from build123d import *

# Parameters (mm, degrees)
F0_W     = 9.2
F0_H     = 5
F1_DEPTH = 8
F3_R     = 0.75
F6_DEPTH = 30
F7_DEPTH = 4.2
F8_DEPTH = 25


with BuildPart() as f1:
    # F0 (on Front) → F1 (new body, symmetric)
    with BuildSketch(Plane.XZ):
        Polygon((-6, -2.5), (-4.6, -2.5), (-4.6, 2.5), align=None)
        Rectangle(F0_W, F0_H)
        Polygon((4.6, -2.5), (6, -2.5), (4.6, 2.5), align=None)
    extrude(amount=F1_DEPTH, both=True)

    # F3
    f3_edges = [f1.edges().sort_by_distance(p)[0] for p in [
        (-4.6, 0, 2.5),
        (4.6, 0, 2.5),
        (6, 0, -2.5),
        (-6, 0, -2.5),
    ]]
    fillet(f3_edges, radius=F3_R)

    # F5 (on face) → F6 (cut)
    with BuildSketch(Plane.XZ.offset(8)):
        with BuildLine():
            Line((7.368007, 1), (7.368007, 4))
            Line((7.368007, 4), (-7.368007, 4))
            Line((-7.368007, 4), (-7.368007, 1))
            Line((-7.368007, 1), (-5.02, 1))
            Line((-5.02, 1), (-4.753378, 1.952222))
            ThreePointArc((-4.753378, 1.952222), (-4.484384, 2.347565), (-4.031155, 2.5))
            Line((-4.031155, 2.5), (4.031155, 2.5))
            ThreePointArc((4.031155, 2.5), (4.484384, 2.347565), (4.753378, 1.952222))
            Line((4.753378, 1.952222), (5.02, 1))
            Line((5.02, 1), (7.368007, 1))
        make_face()
        with BuildLine():
            Line((-5.02, 1), (5.02, 1))
            Line((5.02, 1), (4.753378, 1.952222))
            ThreePointArc((4.753378, 1.952222), (4.484384, 2.347565), (4.031155, 2.5))
            Line((4.031155, 2.5), (-4.031155, 2.5))
            ThreePointArc((-4.031155, 2.5), (-4.484384, 2.347565), (-4.753378, 1.952222))
            Line((-4.753378, 1.952222), (-5.02, 1))
        make_face()
    extrude(amount=-F6_DEPTH, mode=Mode.SUBTRACT)

    # F4 (on face) → F7 (cut)
    with BuildSketch(Plane.XY.offset(2.5)):
        Polygon((3.95, -2.280534), (3.95, 2.280534), (0, 4.561067), (-3.95, 2.280534), (-3.95, -2.280534), (0, -4.561067), align=None)
    extrude(amount=-F7_DEPTH, mode=Mode.SUBTRACT)

    # F2 (on face) → F8 (cut)
    with BuildSketch(Plane(origin=(0, 0, -2.5), x_dir=(1, 0, 0), z_dir=(0, 0, -1))):
        with BuildLine():
            Line((0, -2), (0, 0))
            Line((0, 0), (0, 2))
            ThreePointArc((0, 2), (-2, 0), (0, -2))
        make_face()
        with BuildLine():
            Line((0, 2), (0, 0))
            Line((0, 0), (0, -2))
            ThreePointArc((0, -2), (1.414214, -1.414214), (2, 0))
            ThreePointArc((2, 0), (1.414214, 1.414214), (0, 2))
        make_face()
    extrude(amount=-F8_DEPTH, mode=Mode.SUBTRACT)


solid = f1.part
Input: part model. Units: mm. Frame: model coordinates. A direction names the side the tool comes from. Round coordinates to 2 decimals unless told otherwise and drop trailing zeros. Order: outer loops, then holes, each group sorted by start corner. A loop starts at its lowest first (then second) coordinate and runs counter-clockwise, first axis right, second up. Notation, with made-up numbers: (78, -29) - (132, -29) arc R20 cw to (132, -9) - close; hole circle Ø7 at (51, 42.5). An arc over 180 degrees is marked (long way). Use a Markdown table: item, result.
1. Mould query, pull axis Y, two halves, no side actions, for faces 1 (the face through (-1.947, 3.437, -0.331)), 2 (the face through (0, 8, -1)), 3 (the face through (-5.372, -0.112, -0.256)). Classes: +Y half, -Y half, draft (parallel to the pull), parting line (faces both ways), or undercut.
Evaluation:
| item | result |
|---|---|
| face 1 | undercut |
| face 2 | +Y half |
| face 3 | draft |
2. Section A-A on x = -1.75. Return the cut outline in (y, z).
Evaluation:
| item | result |
|---|---|
| outline | (-8, -2.5) - (-0.97, -2.5) - (-0.97, -1.7) - (-3.55, -1.7) - (-3.55, 1) - (-8, 1) - close; (0.97, -2.5) - (8, -2.5) - (8, 1) - (3.55, 1) - (3.55, -1.7) - (0.97, -1.7) - close |
3. Section D-D on y = -6. Return the cut outline in (x, z).
Evaluation:
| item | result |
|---|---|
| outline | (-5.73, -1.55) arc R0.75 ccw to (-5.01, -2.5) - (5.01, -2.5) arc R0.75 ccw to (5.73, -1.55) - (5.02, 1) - (-5.02, 1) - close |
4. Section B-B on z = -0.5. Return the cut outline in (x, y), then the cut area to 3 significant figures.
Evaluation:
| item | result |
|---|---|
| outline | (-5.44, -8) - (5.44, -8) - (5.44, 8) - (-5.44, 8) - close; hole (-3.95, -2.28) - (0, -4.56) - (3.95, -2.28) - (3.95, 2.28) - (0, 4.56) - (-3.95, 2.28) - close |
| area | 120 mm^2 |
5. Section C-C on y = 1.75. Return the cut outline in (x, z).
Evaluation:
| item | result |
|---|---|
| outline | (-5.73, -1.55) arc R0.75 ccw to (-5.01, -2.5) - (-0.97, -2.5) - (-0.97, -1.7) - (-3.95, -1.7) - (-3.95, 1) - (-5.02, 1) - close; (0.97, -2.5) - (5.01, -2.5) arc R0.75 ccw to (5.73, -1.55) - (5.02, 1) - (3.95, 1) - (3.95, -1.7) - (0.97, -1.7) - close |
6. Material intervals for probe 1 along Z at (x, y) = (-2.5, 0.5); probe 2 along Y at (x, z) = (-2, 0.5); probe 3 along X at (y, z) = (3.25, -1.1), sorted ascending.
Evaluation:
| item | result |
|---|---|
| probe 1 | -2.5 to -1.7 |
| probe 2 | -8 to -3.41, 3.41 to 8 |
| probe 3 | -5.61 to -2.27, 2.27 to 5.61 |
7. First-contact query: pin 1 (0.8 mm diameter, centred on y = 0.5, z = -1, fed in from +X); pin 2 (2 mm diameter, centred on y = 0, z = -1, fed in from -X); pin 3 (2.5 mm diameter, centred on x = -1, y = 1.5, fed in from +Z). Flat tips, straight axial feed; report the tip coordinate or a pass-through.
Evaluation:
| item | result |
|---|---|
| pin 1 | x = 5.69 |
| pin 2 | x = -5.76 |
| pin 3 | z = -1.7 |
8. Access query for faces 4 (the face through (-2.003, -3.405, -0.331)), 5 (the face through (0, -8, -1)). Directions: +Z, -Z, +X, -X, +Y, -Y. A direction counts if a zero-diameter tool reaches every point of the face in a straight line with its end or side. Return the directions, or none.
Evaluation:
| item | result |
|---|---|
| face 4 | +Z |
| face 5 | +Z, -Z, +X, -X, -Y |
